Input: part model. Units: mm. Frame: model coordinates. A direction names the side the tool comes from. Coordinates: 2 decimals unless noted, no trailing zeros. Order: outer loops, then holes, each group sorted by start corner. A loop starts at its lowest first (then second) coordinate and runs counter-clockwise, first axis right, second up. Notation, with made-up numbers: M 85.25,41 L 115.25,41 A29 cw 115.25,73 Z; hole C 86,42.25 d11. An arc over 180 degrees is marked long. Answer in a Markdown table with one row per item.
from build123d import *

# Parameters (mm, degrees)
SKETCH1_R          = 27
SKETCH1_R_2        = 18.25
EXTRUDE1_DEPTH     = 8
CUT_EXTRUDE1_DEPTH = 9
CIRPATTERN1_COUNT  = 4


with BuildPart() as part:
    # Sketch1 → Extrude1 (new body)
    with BuildSketch(Plane.XY):
        Circle(SKETCH1_R)
        Circle(SKETCH1_R_2, mode=Mode.SUBTRACT)
    extrude(amount=EXTRUDE1_DEPTH)

    # Sketch2 → Cut-Extrude1 (cut, through all)
    with BuildSketch(Plane.XY.offset(8)):
        with BuildLine():
            Line((16.455921283, 21.405668752), (14.28355698, 19.233304448))
            Line((14.28355698, 19.233304448), (19.233304448, 14.28355698))
            Line((19.233304448, 14.28355698), (21.405668752, 16.455921283))
            ThreePointArc((21.405668752, 16.455921283), (19.091883092, 19.091883092), (16.455921283, 21.405668752))
        make_face()
    cut_extrude1 = extrude(amount=-CUT_EXTRUDE1_DEPTH, mode=Mode.SUBTRACT)

    # CirPattern1: Cut-Extrude1 ×4 about axis
    cirpattern1_axis = Axis((0, 0, 0), (0, 0, 1))
    for i in range(1, CIRPATTERN1_COUNT):
        add(cut_extrude1.rotate(cirpattern1_axis, i * 360 / CIRPATTERN1_COUNT), mode=Mode.SUBTRACT)

    # Sketch3 → Cut-Revolve1 (revolve, cut)
    with BuildSketch(Plane(origin=(0, 0, 0), x_dir=(1, 0, 0), z_dir=(0, 1, 0))):
        Polygon((27, 0), (23.5, 0), (27, -2.272926576), align=None)
    revolve(axis=Axis((0, 0, 0), (0, 0, -1)), mode=Mode.SUBTRACT)


solid = part.part
1) Cut plane B-B, the plane z = 7.25. Output: boundary loops of the cut face in (x, y).
Resolved:
| item | result |
|---|---|
| outline | M -21.41,-16.46 L -19.23,-14.28 L -14.28,-19.23 L -16.46,-21.41 A27 ccw 16.46,-21.41 L 14.28,-19.23 L 19.23,-14.28 L 21.41,-16.46 A27 ccw 21.41,16.46 L 19.23,14.28 L 14.28,19.23 L 16.46,21.41 A27 ccw -16.46,21.41 L -14.28,19.23 L -19.23,14.28 L -21.41,16.46 A27 ccw Z; hole C 0,0 d36.5 |
2) Contact query for flat-ended pins moving along their axis: pin 1 (4 mm diameter, centred on y = -14, z = 1.5, fed in from -X); pin 2 (3 mm diameter, centred on x = 4, y = -21, fed in from -Z); pin 3 (1 mm diameter, centred on y = -3, z = 4, fed in from +X). Output: stop coordinate, or through.
Resolved:
| item | result |
|---|---|
| pin 1 | stops at x = -24.11 |
| pin 2 | stops at z = 0 |
| pin 3 | stops at x = 26.88 |
3) Mould query, pull axis X, two halves, no side actions, for faces 6 (the face through (-27, 0, 5)), 7 (the face through (-16.724, -16.793, 4.12)), 8 (the face through (15.38, 20.33, 5.06)). Classes: +X half, -X half, draft (parallel to the pull), parting line (faces both ways), or undercut.
Resolved:
| item | result |
|---|---|
| face 6 | -X half |
| face 7 | undercut |
| face 8 | +X half |
4) Cut plane A-A, the plane x = 0. Output: boundary loops of the cut face in (y, z), and give its area (3 significant figures).
Resolved:
| item | result |
|---|---|
| outline | M -27,2.27 L -23.5,0 L -18.25,0 L -18.25,8 L -27,8 Z; M 18.25,0 L 23.5,0 L 27,2.27 L 27,8 L 18.25,8 Z |
| area | 132 mm2 |
5) Reachability of faces 1 (the face through (20.33, -15.38, 5.06)), 2 (the face through (-15.35, 20.3, 5.06)), 3 (the face through (16.724, 16.793, 4.12)), 4 (the face through (15.35, -20.3, 5.06)), 5 (the face through (21.91, 9.08, 0.14)) from +Z, -Z, +X, -X, +Y, -Y: full face, straight path, thin tool, end or side. Return the list, or none.
Resolved:
| item | result |
|---|---|
| face 1 | +Z, -Z, -Y |
| face 2 | +Z, -Z, -X |
| face 3 | +Z, -Z |
| face 4 | +Z, -Z, +X |
| face 5 | -Z |
6) Material intervals for probe 1 along Y at (x, z) = (0, 2.5); probe 2 along X at (y, z) = (-14.5, 6.5); probe 3 along X at (y, z) = (15.5, 4.5), sorted ascending.
Resolved:
| item | result |
|---|---|
| probe 1 | y = -27 to -18.25, 18.25 to 27 |
| probe 2 | x = -22.78 to -19.45, -19.02 to -11.08, 11.08 to 19.02, 19.45 to 22.78 |
| probe 3 | x = -22.11 to -20.45, -18.02 to -9.63, 9.63 to 18.02, 20.45 to 22.11 |
